```python
from build123d import *

# Parameters (mm, degrees)
F1_DEPTH = 228.6


with BuildPart() as f1:
    # F0 (on Front) → F1 (new body, symmetric)
    with BuildSketch(Plane.XZ):
        with BuildLine():
            ThreePointArc((-1.5875, 0), (-1.122532, 1.122532), (0, 1.5875))
            Line((0, 1.5875), (-330.2, 1.5875))
            Line((-330.2, 1.5875), (-330.2, 0))
            Line((-330.2, 0), (-1.5875, 0))
        make_face()
        with BuildLine():
            Line((1.5875, -38.1), (1.5875, 0))
            ThreePointArc((1.5875, 0), (1.122532, -1.122532), (0, -1.5875))
            Line((0, -1.5875), (0, -38.1))
            Line((0, -38.1), (1.5875, -38.1))
        make_face()
        with BuildLine():
            ThreePointArc((0, -1.5875), (1.122532, -1.122532), (1.5875, 0))
            ThreePointArc((1.5875, 0), (1.122532, 1.122532), (0, 1.5875))
            ThreePointArc((0, 1.5875), (-1.122532, 1.122532), (-1.5875, 0))
            ThreePointArc((-1.5875, 0), (-1.122532, -1.122532), (0, -1.5875))
        make_face()
    extrude(amount=F1_DEPTH, both=True)


solid = f1.part
```
Here's how the part is built. I have some questions about the finished solid (model axes, mm). A direction names the side the tool comes from. Coordinates: 2 decimals unless noted, no trailing zeros. Loops run counter-clockwise (first coordinate to the right, second up) from the corner with the lowest first, then second, coordinate; pieces in that order, holes last. Notation, with made-up numbers: M -15.75,-26 L -11.75,-26 A16 ccw -11.75,-7 Z; hole C 57,72 d7. An arc over 180 degrees is marked long. One line per item, written item: value.
1. On a 3-axis mill with a long thin cutter (end or side, diameter ignored), from which of +Z, -Z, +X, -X, +Y, -Y can I reach the whole of each face in a straight line? I mean faces 1 (the flat face through (-168, -3, 0)), 2 (the flat face through (-165, -228.6, 1)). Say none if no direction works.
Geometry says:
face 1: -Z, -X, +Y, -Y
face 2: +Z, -Z, +X, -X, -Y
2. Please list where these lines run through material, in increasing order: probe 1 along Z at (x, y) = (-96.5, 58.5); probe 2 along X at (y, z) = (-194.5, -1).
Geometry says:
probe 1: z = 0 to 1.59
probe 2: x = -1.23 to 1.59
3. Imagine slicing it at A-A (y = -166.5). List the corners of the cut face in (x, z) for me (1 decimal).
Geometry says:
outline: M -330.2,0 L -1.6,0 A1.6 ccw 0,-1.6 L 0,-38.1 L 1.6,-38.1 L 1.6,0 A1.6 ccw 0,1.6 L -330.2,1.6 Z
4. Imagine slicing it at C-C (z = -13). List the corners of the cut face in (x, y) for me.
Geometry says:
outline: M 0,-228.6 L 1.59,-228.6 L 1.59,228.6 L 0,228.6 Z
5. Will these pins go through, and if not, where does the flat tip stop? pin 1 Ø6 at (y, z) = (-42.5, -3.5) entering from -X; pin 2 Ø8 at (x, y) = (-288.5, -81) entering from -Z; pin 3 Ø1 at (y, z) = (-136.5, -20.5) entering from -X.
Geometry says:
pin 1: stops at x = -1.51
pin 2: stops at z = 0
pin 3: stops at x = 0
6. Imagine slicing it at B-B (x = -177.5). List the corners of the cut face in (y, z) for me, and give its area (3 significant figures).
Geometry says:
outline: M -228.6,0 L 228.6,0 L 228.6,1.59 L -228.6,1.59 Z
area: 726 mm2
